CAD build for the part. Positions are in the model's coordinates, mm. Face numbers are marked on the shaded views. A direction names the side the tool comes from. Round coordinates to 2 decimals unless told otherwise and drop trailing zeros. Loops run counter-clockwise (first coordinate to the right, second up) from the corner with the lowest first, then second, coordinate; pieces in that order, holes last.
from build123d import *

# Parameters (mm, degrees)
SKETCH1_W           = 31.9
SKETCH1_H           = 34
BOSS_EXTRUDE3_DEPTH = 2
SKETCH2_W           = 4.7
SKETCH2_H           = 22
BOSS_EXTRUDE4_DEPTH = 25
SKETCH3_W           = 22.5
SKETCH3_H           = 2
SKETCH3_W_2         = 31.9
BOSS_EXTRUDE5_DEPTH = 4
SKETCH6_W           = 27.2
SKETCH6_H           = 2.5
SKETCH6_W_2         = 4.7
CUT_EXTRUDE1_DEPTH  = 11.8
SKETCH7_R           = 0.65
CUT_EXTRUDE2_DEPTH  = 4
BOSS_EXTRUDE6_DEPTH = 10


with BuildPart() as part:
    # Sketch1 → Boss-Extrude3 (new body)
    with BuildSketch(Plane(origin=(0, 0, 0), x_dir=(1, 0, 0), z_dir=(0, 1, 0))):
        Rectangle(SKETCH1_W, SKETCH1_H)
    extrude(amount=BOSS_EXTRUDE3_DEPTH)

    # Sketch2 → Boss-Extrude4 (add)
    with BuildSketch(Plane(origin=(0, 2, 0), x_dir=(1, 0, 0), z_dir=(0, 1, 0))):
        with Locations((-13.6, 6)):
            Rectangle(SKETCH2_W, SKETCH2_H)
        with Locations((13.6, 6)):
            Rectangle(SKETCH2_W, SKETCH2_H)
    extrude(amount=BOSS_EXTRUDE4_DEPTH)

    # Sketch3 → Boss-Extrude5 (add)
    with BuildSketch(Plane(origin=(0, 2, 0), x_dir=(1, 0, 0), z_dir=(0, 1, 0))):
        with Locations((0, -4)):
            Rectangle(SKETCH3_W, SKETCH3_H)
        with Locations((0, -16)):
            Rectangle(SKETCH3_W_2, SKETCH3_H)
    extrude(amount=BOSS_EXTRUDE5_DEPTH)

    # Sketch6 → Cut-Extrude1 (cut)
    with BuildSketch(Plane(origin=(0, 27, 0), x_dir=(1, 0, 0), z_dir=(0, 1, 0))):
        with Locations((2.35, -0.15)):
            Rectangle(SKETCH6_W, SKETCH6_H)
        with Locations((-13.6, -0.15)):
            Rectangle(SKETCH6_W_2, SKETCH6_H)
    extrude(amount=-CUT_EXTRUDE1_DEPTH, mode=Mode.SUBTRACT)

    # Sketch7 → Cut-Extrude2 (cut)
    with BuildSketch(Plane.XY.offset(5)):
        with Locations((-13.6, 21.1)):
            Circle(SKETCH7_R)
        with Locations((13.6, 21.1)):
            Circle(SKETCH7_R)
    extrude(amount=-CUT_EXTRUDE2_DEPTH, mode=Mode.SUBTRACT)

    # Sketch8 → Boss-Extrude6 (add)
    with BuildSketch(Plane(origin=(0, 0, 0), x_dir=(1, 0, 0), z_dir=(0, 1, 0))):
        Polygon((5.95, -65), (15.95, -56.609003688), (15.95, -17), (5.95, -17), align=None)
    extrude(amount=BOSS_EXTRUDE6_DEPTH)


solid = part.part
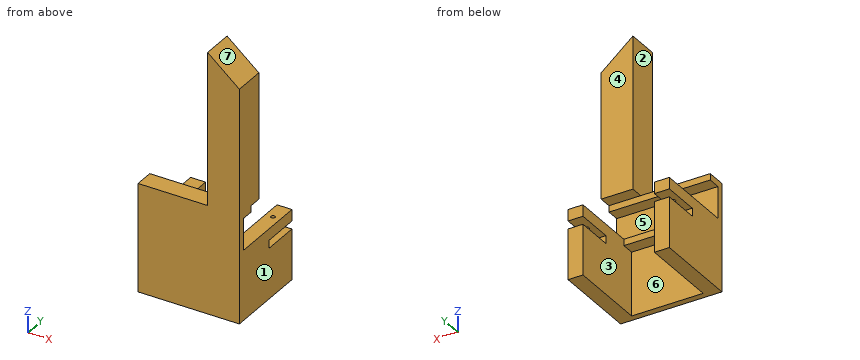
Item 1: Flat gauge pins, fed straight in: P1, Ø2, axis at x = -4, z = 16, coming from the +Y side; P2, Ø6, axis at x = 4.5, z = 45.5, coming from the +Y side; P3, Ø10, axis at x = -10.5, y = 5, coming from the +Z side. Where does each tip first touch, or does it go through?
Verdict:
P1: stops at y = 6
P2: stops at y = 10
P3: stops at z = 17
Item 2: Cut at B-B (x = 5). List the corners of the cut face in (y, z), plus the area to 3 significant figures.
Verdict:
outline: (0, -17) - (2, -17) - (2, 3) - (6, 3) - (6, 5) - (2, 5) - (2, 15) - (6, 15) - (6, 17) - (0, 17) - close
area: 84.0 mm2
Item 3: Cut at D-D (z = -8). List the corners of the cut face in (x, y), plus the area to 3 significant figures.
Verdict:
outline: (-15.95, 0) - (15.95, 0) - (15.95, 27) - (11.25, 27) - (11.25, 2) - (-11.25, 2) - (-11.25, 27) - (-15.95, 27) - close
area: 299 mm2
Item 4: Cut at A-A (y = 22.5). List the corners of the cut face in (x, z), plus the area to 3 significant figures.
Verdict:
outline: (-15.95, -17) - (-11.25, -17) - (-11.25, -1.1) - (-15.95, -1.1) - close; (-15.95, 1.4) - (-11.25, 1.4) - (-11.25, 5) - (-15.95, 5) - close; (11.25, -17) - (15.95, -17) - (15.95, -1.1) - (11.25, -1.1) - close; (11.25, 1.4) - (15.95, 1.4) - (15.95, 5) - (11.25, 5) - close
area: 183 mm2
Item 5: Cut at C-C (y = 6.75). List the corners of the cut face in (x, z), plus the area to 3 significant figures.
Verdict:
outline: (-15.95, -17) - (-11.25, -17) - (-11.25, 5) - (-15.95, 5) - close; (5.95, 17) - (15.95, 17) - (15.95, 56.61) - (5.95, 65) - close; (11.25, -17) - (15.95, -17) - (15.95, 5) - (11.25, 5) - close
area: 645 mm2
Item 6: Mould opens along Z. For the marked faces 5, 6 and 7 say: released by +Z, released by -Z, zero draft, split by the parting line, or undercut.
Verdict:
face 5: undercut
face 6: zero draft
face 7: released by +Z
Item 7: Wall check: L1, parallel to Z at x = -13, y = 24.25; L2, parallel to Y at x = -13.6, z = 3.05; L3, parallel to X at y = 21, z = -11.5. Give the ranges that are in metal, low to high.
Verdict:
L1: z = -17 to -1.1, 1.4 to 5
L2: y = 0 to 20.45, 21.75 to 27
L3: x = -15.95 to -11.25, 11.25 to 15.95
Item 8: 3-axis set-ups, long thin cutter, end or side, ignore diameter. For the marked faces 1, 2, 3 and 4: which of +Z, -Z, +X, -X, +Y, -Y reach the whole face in a straight line?
Verdict:
face 1: +Z, -Z, +X, +Y, -Y
face 2: +Z, -X, +Y, -Y
face 3: -Z, +Y
face 4: +Z, +X, -X, +Y
